```python
from build123d import *

# Parameters (mm, degrees)
SKETCH_1_W           = 20
SKETCH_1_H           = 20
EXTRUDE_1_DEPTH      = 120
SKETCH_2_W           = 10
SKETCH_2_H           = 20
CUT_EXTRUDE_1_DEPTH  = 120
CUT_EXTRUDE_2_DEPTH  = 120
SKETCH_4_R           = 3
CUT_EXTRUDE_3_DEPTH  = 2
SKETCH_6_R           = 1.49
CUT_EXTRUDE_4_DEPTH  = 20
CUT_EXTRUDE_5_DEPTH  = 20
SKETCH_8_W           = 19.6
SKETCH_8_H           = 0.2
SKETCH_8_W_2         = 0.2
SKETCH_8_H_2         = 19.6
CUT_EXTRUDE_6_DEPTH  = 45
EXTRUDE_2_DEPTH      = 24.8
EXTRUDE_START        = 5.2
EXTRUDE_3_DEPTH      = 5.2
SKETCH_12_W          = 20
SKETCH_12_H          = 20
EXTRUDE_4_DEPTH      = 15
SKETCH_13_W          = 5
SKETCH_13_H          = 5
SKETCH_13_H_2        = 4.5
CUT_EXTRUDE_8_DEPTH  = 15
SKETCH_14_R          = 2
CUT_EXTRUDE_9_DEPTH  = 70
SKETCH_15_W          = 10
SKETCH_15_H          = 5.5
CUT_EXTRUDE_10_DEPTH = 15
CUT_EXTRUDE_11_DEPTH = 5
CUT_EXTRUDE_12_DEPTH = 20
SKETCH_18_R          = 3
CUT_EXTRUDE_13_DEPTH = 2
SKETCH_19_W          = 0.2
SKETCH_19_H          = 25.5
CUT_EXTRUDE_14_DEPTH = 15
SKETCH_21_W          = 10.4
SKETCH_21_H          = 0.2
CUT_EXTRUDE_15_DEPTH = 15


with BuildPart() as part:
    # 草图1 → 凸台-拉伸1 (new body)
    with BuildSketch(Plane.XY):
        with Locations((10, 10)):
            Rectangle(SKETCH_1_W, SKETCH_1_H)
    extrude(amount=EXTRUDE_1_DEPTH)

    # 草图2 → 切除-拉伸1 (cut)
    with BuildSketch(Plane(origin=(0, 20, 0), x_dir=(1, 0, 0), z_dir=(0, 1, 0))):
        with Locations((15, -10)):
            Rectangle(SKETCH_2_W, SKETCH_2_H)
    extrude(amount=-CUT_EXTRUDE_1_DEPTH, mode=Mode.SUBTRACT)

    # 草图3 → 切除-拉伸2 (cut)
    with BuildSketch(Plane(origin=(10, 0, 0), x_dir=(0, 0, -1), z_dir=(1, 0, 0))):
        with BuildLine():
            ThreePointArc((-8.45, 10), (-9.40684068, 11.432013275), (-11.096015511, 11.096015511))
            Line((-11.096015511, 11.096015511), (-8.903984489, 8.903984489))
            ThreePointArc((-8.903984489, 8.903984489), (-8.567986725, 9.40684068), (-8.45, 10))
        make_face()
        with BuildLine():
            Line((-8.903984489, 8.903984489), (-11.096015511, 11.096015511))
            ThreePointArc((-11.096015511, 11.096015511), (-11.096015511, 8.903984489), (-8.903984489, 8.903984489))
        make_face()
    extrude(amount=-CUT_EXTRUDE_2_DEPTH, mode=Mode.SUBTRACT)

    # 草图4 → 切除-拉伸3 (cut)
    with BuildSketch(Plane.ZY):
        with Locations((10, 10)):
            Circle(SKETCH_4_R)
    extrude(amount=-CUT_EXTRUDE_3_DEPTH, mode=Mode.SUBTRACT)

    # 草图6 → 切除-拉伸4 (cut)
    with BuildSketch(Plane.ZY):
        with Locations((92.5, 10)):
            Circle(SKETCH_6_R)
    extrude(amount=-CUT_EXTRUDE_4_DEPTH, mode=Mode.SUBTRACT)

    # 草图7 → 切除-拉伸5 (cut)
    with BuildSketch(Plane.XZ):
        with BuildLine():
            ThreePointArc((11.55, 97.5), (10.844615988, 98.799662969), (9.370485378, 98.9164079))
            Line((9.370485378, 98.9164079), (10.629514622, 96.0835921))
            ThreePointArc((10.629514622, 96.0835921), (11.299662969, 96.655384012), (11.55, 97.5))
        make_face()
        with BuildLine():
            Line((10.629514622, 96.0835921), (9.370485378, 98.9164079))
            ThreePointArc((9.370485378, 98.9164079), (8.5835921, 96.870485378), (10.629514622, 96.0835921))
        make_face()
    extrude(amount=-CUT_EXTRUDE_5_DEPTH, mode=Mode.SUBTRACT)

    # 草图8 → 切除-拉伸6 (cut)
    with BuildSketch(Plane.XY.offset(120)):
        with Locations((10, 19.9)):
            Rectangle(SKETCH_8_W, SKETCH_8_H)
        with Locations((0.1, 19.9)):
            Rectangle(SKETCH_8_W_2, SKETCH_8_H)
        with Locations((0.1, 10)):
            Rectangle(SKETCH_8_W_2, SKETCH_8_H_2)
        with Locations((19.9, 10)):
            Rectangle(SKETCH_8_W_2, SKETCH_8_H_2)
        with Locations((19.9, 0.1)):
            Rectangle(SKETCH_8_W_2, SKETCH_8_H)
        with Locations((10, 0.1)):
            Rectangle(SKETCH_8_W, SKETCH_8_H)
        with Locations((0.1, 0.1)):
            Rectangle(SKETCH_8_W_2, SKETCH_8_H)
        with Locations((19.9, 19.9)):
            Rectangle(SKETCH_8_W_2, SKETCH_8_H)
    extrude(amount=-CUT_EXTRUDE_6_DEPTH, mode=Mode.SUBTRACT)

    # 草图9 → 凸台-拉伸2 (add)
    with BuildSketch(Plane(origin=(0, 19.8, 0), x_dir=(1, 0, 0), z_dir=(0, 1, 0))):
        with BuildLine():
            Line((0, -75), (-10, -75))
            ThreePointArc((-10, -75), (-2.928932188, -77.928932188), (0, -85))
            Line((0, -85), (0.2, -85))
            Line((0.2, -85), (0.2, -75))
            Line((0.2, -75), (0, -75))
        make_face()
    extrude(amount=-EXTRUDE_2_DEPTH)

    # 草图10 → 凸台-拉伸3 (add)
    with BuildSketch(Plane(origin=(0, 19.8, 0), x_dir=(1, 0, 0), z_dir=(0, 1, 0)).offset(EXTRUDE_START)):
        with BuildLine():
            Line((-10, -75), (0, -75))
            Line((0, -75), (0.2, -75))
            Line((0.2, -75), (0.2, -85))
            Line((0.2, -85), (0, -85))
            ThreePointArc((0, -85), (-2.928932188, -77.928932188), (-10, -75))
        make_face()
    extrude(amount=-EXTRUDE_3_DEPTH)

    # 草图12 → 凸台-拉伸4 (add)
    with BuildSketch(Plane.XZ):
        with Locations((10, 65)):
            Rectangle(SKETCH_12_W, SKETCH_12_H)
    extrude(amount=EXTRUDE_4_DEPTH)

    # 草图13 → 切除-拉伸8 (cut)
    with BuildSketch(Plane.ZY):
        Polygon((60, 10.5), (60, 0), (65, 0), (70, 0), (70, 10.5), align=None)
        with Locations((62.5, -2.5)):
            Rectangle(SKETCH_13_W, SKETCH_13_H)
        with Locations((67.5, -2.5)):
            Rectangle(SKETCH_13_W, SKETCH_13_H)
        with Locations((62.5, -7.25)):
            Rectangle(SKETCH_13_W, SKETCH_13_H_2)
        with Locations((67.5, -7.25)):
            Rectangle(SKETCH_13_W, SKETCH_13_H_2)
    extrude(amount=-CUT_EXTRUDE_8_DEPTH, mode=Mode.SUBTRACT)

    # 草图14 → 切除-拉伸9 (cut)
    with BuildSketch(Plane(origin=(0, 0, 0), x_dir=(-1, 0, 0), z_dir=(0, 0, -1))):
        with Locations((-5, 14)):
            Circle(SKETCH_14_R)
    extrude(amount=-CUT_EXTRUDE_9_DEPTH, mode=Mode.SUBTRACT)

    # 草图15 → 切除-拉伸10 (cut)
    with BuildSketch(Plane.ZY):
        with Locations((65, 13.25)):
            Rectangle(SKETCH_15_W, SKETCH_15_H)
    extrude(amount=-CUT_EXTRUDE_10_DEPTH, mode=Mode.SUBTRACT)

    # 草图16 → 切除-拉伸11 (cut)
    with BuildSketch(Plane.ZY.offset(-15)):
        with BuildLine():
            ThreePointArc((66.48, 5.5), (65, 6.98), (63.52, 5.5))
            Line((63.52, 5.5), (65, 5.5))
            Line((65, 5.5), (65, 4.02))
            ThreePointArc((65, 4.02), (66.046518036, 4.453481964), (66.48, 5.5))
        make_face()
        with BuildLine():
            Line((65, 5.5), (63.52, 5.5))
            ThreePointArc((63.52, 5.5), (63.953481964, 4.453481964), (65, 4.02))
            Line((65, 4.02), (65, 5.5))
        make_face()
    extrude(amount=-CUT_EXTRUDE_11_DEPTH, mode=Mode.SUBTRACT)

    # 草图17 → 切除-拉伸12 (cut)
    with BuildSketch(Plane.ZY):
        with BuildLine():
            Line((55, -10), (55, -15))
            Line((55, -15), (60, -15))
            ThreePointArc((60, -15), (56.464466094, -13.535533906), (55, -10))
        make_face()
        with BuildLine():
            ThreePointArc((75, -10), (73.535533906, -13.535533906), (70, -15))
            Line((70, -15), (75, -15))
            Line((75, -15), (75, -10))
        make_face()
    extrude(amount=-CUT_EXTRUDE_12_DEPTH, mode=Mode.SUBTRACT)

    # 草图18 → 切除-拉伸13 (cut)
    with BuildSketch(Plane(origin=(20, 0, 0), x_dir=(0, 0, -1), z_dir=(1, 0, 0))):
        with Locations((-65, 5.5)):
            Circle(SKETCH_18_R)
    extrude(amount=-CUT_EXTRUDE_13_DEPTH, mode=Mode.SUBTRACT)

    # 草图19 → 切除-拉伸14 (cut)
    with BuildSketch(Plane.ZY):
        with Locations((70.1, 3.25)):
            Rectangle(SKETCH_19_W, SKETCH_19_H)
        with Locations((59.9, 3.25)):
            Rectangle(SKETCH_19_W, SKETCH_19_H)
    extrude(amount=-CUT_EXTRUDE_14_DEPTH, mode=Mode.SUBTRACT)

    # 草图21 → 切除-拉伸15 (cut)
    with BuildSketch(Plane.ZY):
        with Locations((65, -9.6)):
            Rectangle(SKETCH_21_W, SKETCH_21_H)
    extrude(amount=-CUT_EXTRUDE_15_DEPTH, mode=Mode.SUBTRACT)


solid = part.part
```
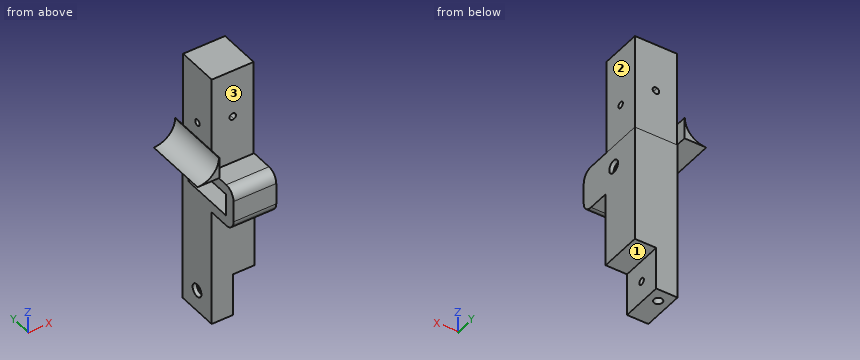
Design review of the part built by this model. Coordinates are the model's own, in mm. Face numbers are marked on the shaded views. A direction names the side the tool comes from. Give positions to 0.01 mm unless a question says otherwise; leave off trailing zeros. Loops run counter-clockwise (first coordinate to the right, second up) from the corner with the lowest first, then second, coordinate; pieces in that order, holes last. Notation, with made-up numbers: (-31, 83) -> (9, 83) arc R14 cw to (9, 91) -> close; hole circle Ø9 at (84, 75). An arc over 180 degrees is marked (long way). Write each question's results on one line, items separated by ' | '.
Q1. Take a section at B-B, the plane z = 92.5. Write out the cut boundary in (x, y), plus the area to 3 significant figures.
Reply:
outline: (0.2, 0.2) -> (19.8, 0.2) -> (19.8, 8.51) -> (0.2, 8.51) -> close; (0.2, 11.49) -> (19.8, 11.49) -> (19.8, 19.8) -> (0.2, 19.8) -> close | area: 326 mm²
Q2. Take a section at D-D, the plane x = -4.75. Write out the cut boundary in (y, z).
Reply:
outline: (-5, 75) -> (25, 75) -> (25, 76.49) -> (-5, 76.49) -> close
Q3. Wall thickness on L1, parallel to Y at x = 15.5, z = 92.5; L2, parallel to X at y = 14, z = 23; L3, parallel to Y at x = 1.55, z = 10: over which ranges is each line inside the solid? List them lowest first.
Reply:
L1: y = 0.2 to 8.51, 11.49 to 19.8 | L2: x = 0 to 3, 7 to 20 | L3: y = 0 to 7, 13 to 20
Q4. Take a section at C-C, the plane x = 13.75. Write out the cut boundary in (y, z).
Reply:
outline: (-15, 60) arc R5 ccw to (-10, 55) -> (0, 55) -> (0, 20) -> (20, 20) -> (20, 75) -> (19.8, 75) -> (19.8, 120) -> (0.2, 120) -> (0.2, 75) -> (-10, 75) arc R5 ccw to (-15, 70) -> close; hole (-9.7, 59.8) -> (16, 59.8) -> (16, 70.2) -> (-9.7, 70.2) -> close; hole circle Ø2.98 at (10, 92.5)
Q5. Machinability: for the marked faces 1, 2 and 3, which of the approach directions +Z, -Z, +X, -X, +Y, -Y give a long, thin tool a straight path to every point of the face, cutting with its end or side? Answer none if there is none.
Reply:
face 1: -Z, +X, +Y, -Y | face 2: +Z, +X, +Y, -Y | face 3: +Z, +X, -Y
Q6. For pin 1 Ø10 at (x, z) = (8, 99) entering from -Y; pin 2 Ø12 at (y, z) = (4, 100.5) entering from +X; pin 3 Ø1 at (x, z) = (6, 42) entering from -Y, all flat-tipped, find the tip position at first contact; note any pin that passes through.
Reply:
pin 1: stops at y = 0.2 | pin 2: stops at x = 19.8 | pin 3: stops at y = 0
Q7. Take a section at A-A, the plane z = 10. Write out the cut boundary in (x, y), plus the area to 3 significant figures.
Reply:
outline: (0, 0) -> (10, 0) -> (10, 8.45) -> (2, 8.45) -> (2, 7) -> (0, 7) -> close; (0, 13) -> (2, 13) -> (2, 11.55) -> (10, 11.55) -> (10, 20) -> (0, 20) -> close; hole circle Ø4 at (5, 14) | area: 151 mm²
